Source: CAD feature listing. Evaluate the final solid. Frame: model axes, mm. Give positions to 0.01 mm unless a question says otherwise; leave off trailing zeros. Loops run counter-clockwise (first coordinate to the right, second up) from the corner with the lowest first, then second, coordinate; pieces in that order, holes last. Notation, with made-up numbers: (-28, -9) -> (9, -9) arc R18 cw to (9, 8) -> close; hole circle Ø3 at (17.5, 10). An arc over 180 degrees is marked (long way). Put each result on its own line as item: value.
```python
from build123d import *


with BuildPart() as part:
    # Sketch1 → Revolve1 (revolve)
    with BuildSketch(Plane(origin=(0, 0, 0), x_dir=(1, 0, 0), z_dir=(0, 1, 0)), mode=Mode.PRIVATE) as revolve1_sk:
        with BuildLine():
            Line((-10.83902439, 12), (-10.83902439, 9.979177887))
            Line((-10.83902439, 9.979177887), (-9.99958636, 9.979177887))
            ThreePointArc((-9.99958636, 9.979177887), (-10.508608574, 9.208564683), (-10.540029762, 8.285547331))
            Line((-10.540029762, 8.285547331), (-9.752554563, 6.222546257))
            ThreePointArc((-9.752554563, 6.222546257), (-8.141995388, 3.29472213), (-7.584446232, 0))
            Line((-7.584446232, 0), (-2.83902439, 0))
            Line((-2.83902439, 0), (-2.83902439, 7.780487805))
            ThreePointArc((-2.83902439, 7.780487805), (-3.78199768, 10.05702671), (-6.058536585, 11))
            Line((-6.058536585, 11), (-8.83902439, 11))
            Line((-8.83902439, 11), (-8.83902439, 12))
            Line((-8.83902439, 12), (-10.83902439, 12))
        make_face()
    revolve(revolve1_sk.sketch.rotate(Axis((0, 0, 0), (1, 0, 0)), 180), axis=Axis((0, 0, 0), (1, 0, 0)))


solid = part.part
```
(1) Section C-C on x = -4.25. Return loops of the section in (y, z), then the cut area to 3 significant figures.
Calculated:
outline: circle Ø20.89 at (0, 0)
area: 343 mm²
(2) Section A-A on y = 0. Return loops of the section in (x, z), then the cut area to 3 significant figures.
Calculated:
outline: (-10.84, -12) -> (-8.84, -12) -> (-8.84, -11) -> (-6.06, -11) arc R3.22 ccw to (-2.84, -7.78) -> (-2.84, 7.78) arc R3.22 ccw to (-6.06, 11) -> (-8.84, 11) -> (-8.84, 12) -> (-10.84, 12) -> (-10.84, 9.98) -> (-10, 9.98) arc R1.7 ccw to (-10.54, 8.29) -> (-9.75, 6.22) arc R10.01 cw to (-9.75, -6.22) -> (-10.54, -8.29) arc R1.7 ccw to (-10, -9.98) -> (-10.84, -9.98) -> close
area: 139 mm²
(3) First-contact query: P1, Ø2, axis at x = -6.5, z = 9, coming from the -Y side; P2, Ø1, axis at x = -5, y = -5.5, coming from the -Z side; P3, Ø3, axis at y = -9.5, z = 1.5, coming from the -X side. Flat tips, straight axial feed; report the tip coordinate or a pass-through.
Calculated:
P1: stops at y = -7.55
P2: stops at z = -9.65
P3: stops at x = -10.84
(4) Section D-D on x = -8. Return loops of the section in (y, z).
Calculated:
outline: circle Ø22 at (0, 0); hole circle Ø5.71 at (0, 0)
(5) Line query: probe 1 along Y at (x, z) = (-8.75, 1.5); probe 2 along Y at (x, z) = (-8.5, -1.5); probe 3 along Y at (x, z) = (-4.5, 8.5). Output: solid intervals per line, ascending. Write a range as from..to.
Calculated:
probe 1: y = -10.9..-4.44, 4.44..10.9
probe 2: y = -10.9..-3.9, 3.9..10.9
probe 3: y = -6.33..6.33
(6) Draft query along Z for faces 1 (the flat face through (-8.839, 10, -5)), 2 (the cylindrical face through (-10.413, -2.997, 9.518)), 3 (the cylindrical face through (-7.47, 10.74, -2.38)). Return one class per face: released by +Z, released by -Z, zero draft, split by the parting line, or undercut.
Calculated:
face 1: zero draft
face 2: undercut
face 3: split by the parting line
